Can you work these out from the model? Positions are in its coordinate system, mm. Give positions to 0.01 mm unless a question says otherwise; leave off trailing zeros. Write each loop counter-clockwise with the first axis right and the second up, starting at its lowest first coordinate (ties: lowest second). Pieces come first, ordered by that corner, then holes.
1. I'm going to push a flat-ended pin straight in: pin 1 (2 mm diameter, centred on x = -239.5, z = 14, fed in from +Y). Where does the tip first touch, or does it pass through?
2. If I drill on probe 1 along Z at (x, y) = (-236.75, -98.5); probe 2 along X at (y, z) = (-211.5, 18), over which ranges is the centre line in solid material (lowest first)?
3. Suppose I cut it at A-A (z = 6). Please give me the cut outline in (x, y).
4. Suppose I cut it at B-B (x = -238). Please give me the cut outline in (y, z), and give its area (3 significant figures).
5. Suppose I cut it at C-C (y = 33.5). Please give me the cut outline in (x, z), and give its area (3 significant figures).
Autodesk Inventor part; units mm, degrees
ref_plane "YZ Plane" through (0, 0, 0) normal (1, 0, 0) x (0, 1, 0)
ref_plane "XZ Plane" through (0, 0, 0) normal (0, 1, 0) x (-1, 0, 0)
ref_plane "XY Plane" through (0, 0, 0) normal (0, 0, 1) x (1, 0, 0)
sketch "Sketch1" plane through (0, 0, 0) normal (0, 0, 1) x (1, 0, 0)
  line L0 (-243.8061, 206.1329) -> (-243.8061, -327.2671)
  line L1 (-243.8061, -327.2671) -> (-218.4061, -327.2671)
  line L2 (-218.4061, -327.2671) -> (-218.4061, 206.1329)
  line L3 (-218.4061, 206.1329) -> (-243.8061, 206.1329)
  point P0 (0, 0)
  dimension "d1" = 533.4
  dimension "d9" = 25.4
extrude "Extrusion1" add sketch "Sketch1" along normal blind 25.4
shell "Shell2" thickness 1.5875 removed faces 2 at (-226.8728, -327.2671, 8.4667) at (-235.3394, 206.1329, 8.4667)
properties part number "Frame_FrontConveyorGuide" material "Aluminum-6061"
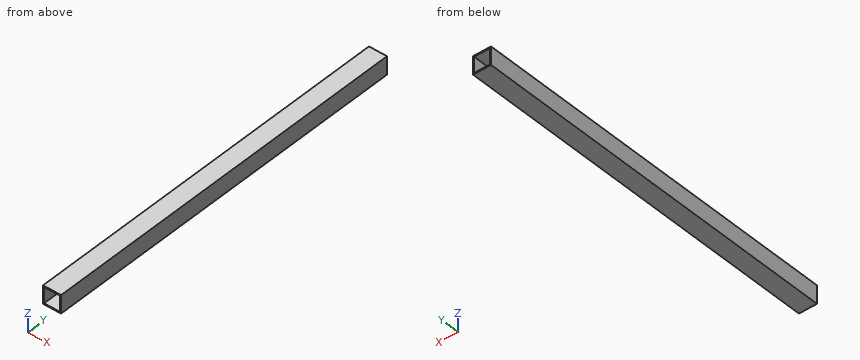
Checks:
1. pin 1: passes through
2. probe 1: z = 0 to 1.59, 23.81 to 25.4
2. probe 2: x = -243.81 to -242.22, -219.99 to -218.41
3. outline: (-243.81, -327.27) - (-242.22, -327.27) - (-242.22, 206.13) - (-243.81, 206.13) - close; (-219.99, -327.27) - (-218.41, -327.27) - (-218.41, 206.13) - (-219.99, 206.13) - close
4. outline: (-327.27, 0) - (206.13, 0) - (206.13, 1.59) - (-327.27, 1.59) - close; (-327.27, 23.81) - (206.13, 23.81) - (206.13, 25.4) - (-327.27, 25.4) - close
4. area: 1,690 mm2
5. outline: (-243.81, 0) - (-218.41, 0) - (-218.41, 25.4) - (-243.81, 25.4) - close; hole (-242.22, 1.59) - (-219.99, 1.59) - (-219.99, 23.81) - (-242.22, 23.81) - close
5. area: 151 mm2
